For this review, take the finished solid that the model builds, in its own axes (mm). Face numbers are marked on the shaded views. A direction names the side the tool comes from. Coordinates: 2 decimals unless noted, no trailing zeros. Write each loop counter-clockwise with the first axis right and the second up, starting at its lowest first coordinate (ties: lowest second). Pieces come first, ordered by that corner, then holes. Notation, with made-up numbers: M 16,70 L 40,70 A13 ccw 40,91 Z; hole C 75.5,49.5 d11. An arc over 180 degrees is marked long. One line per question, with ' | ' between items.
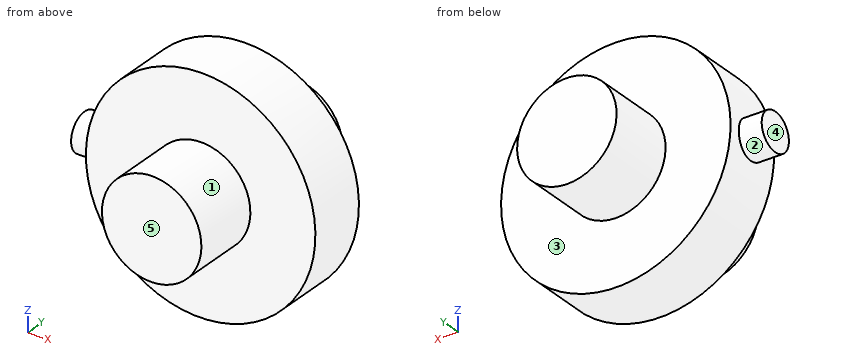
from build123d import *

# Parameters (mm, degrees)
SKETCH1_R           = 5
BOSS_EXTRUDE1_DEPTH = 10
SKETCH2_R           = 30
BOSS_EXTRUDE2_DEPTH = 8
SKETCH3_R           = 13
BOSS_EXTRUDE3_DEPTH = 26


with BuildPart() as part:
    # Sketch1 → Boss-Extrude1 (new body)
    with BuildSketch(Plane(origin=(0, 0, 0), x_dir=(0, 0, -1), z_dir=(1, 0, 0))):
        Circle(SKETCH1_R)
    extrude(amount=BOSS_EXTRUDE1_DEPTH)

    # Sketch2 → Boss-Extrude2 (add, symmetric)
    with BuildSketch(Plane(origin=(0, 0, 0), x_dir=(1, 0, 0), z_dir=(0, 1, 0))):
        with Locations(Location((36, 0, 0), (0, 0, 270))):
            Circle(SKETCH2_R)
    extrude(amount=BOSS_EXTRUDE2_DEPTH, both=True)

    # Sketch3 → Boss-Extrude3 (add, symmetric)
    with BuildSketch(Plane(origin=(0, 0, 0), x_dir=(1, 0, 0), z_dir=(0, 1, 0))):
        with Locations(Location((36, 0, 0), (0, 0, 90))):
            Circle(SKETCH3_R)
    extrude(amount=BOSS_EXTRUDE3_DEPTH, both=True)


solid = part.part
1) Machinability: for the marked faces 1, 2, 3, 4 and 5, which of the approach directions +Z, -Z, +X, -X, +Y, -Y give a long, thin tool a straight path to every point of the face, cutting with its end or side? Answer none if there is none.
Responses:
face 1: -Y | face 2: -X | face 3: +Y | face 4: +Z, -Z, -X, +Y, -Y | face 5: +Z, -Z, +X, -X, -Y
2) We need section D-D on y = 0. State the section outline as (x, z) points.
Responses:
outline: M 0,-5 L 6.42,-5 A30 ccw long 6.42,5 L 0,5 Z
3) To check wall thickness, follow line 1 along X through (y, z) = (0, -1); line 2 along Y through (x, z) = (56, -1); line 3 along Z through (x, y) = (28.5, 22.5). State the ranges of each line that lie inside material, in increasing order. Write a range as [from, to].
Responses:
line 1: [0, 65.98] | line 2: [-8, 8] | line 3: [-10.62, 10.62]
4) Insertion check: pin 1 Ø10 at (y, z) = (13.5, 9.5) entering from -X; pin 2 Ø2 at (x, y) = (34, -19) entering from -Z; pin 3 Ø5 at (x, z) = (29.5, -23.5) entering from +Y. Each pin has a flat end and moves straight along its axis. Give the tip position at first contact, or say it passes through.
Responses:
pin 1: x = 23.8 | pin 2: z = -12.96 | pin 3: y = 8
5) We need section B-B on z = 0. State the section outline as (x, y) points.
Responses:
outline: M 0,-5 L 6,-5 L 6,-8 L 23,-8 L 23,-26 L 49,-26 L 49,-8 L 66,-8 L 66,8 L 49,8 L 49,26 L 23,26 L 23,8 L 6,8 L 6,5 L 0,5 Z
6) We need section A-A on x = 36. State the section outline as (y, z) points.
Responses:
outline: M -26,-13 L -8,-13 L -8,-30 L 8,-30 L 8,-13 L 26,-13 L 26,13 L 8,13 L 8,30 L -8,30 L -8,13 L -26,13 Z
7) We need section C-C on y = -20. State the section outline as (x, z) points.
Responses:
outline: C 36,0 d26
